```python
from build123d import *

# Parameters (mm, degrees)
SKETCH1_W           = 74.93
SKETCH1_H           = 23.368
BOSS_EXTRUDE1_DEPTH = 20.828
SKETCH2_W           = 5.08
SKETCH2_H           = 10.16
SKETCH2_W_2         = 1.27
BOSS_EXTRUDE2_DEPTH = 7.62
FILLET1_R           = 2.54
FILLET2_R           = 3.81
FILLET3_R           = 2.54
FILLET4_R           = 2.54


with BuildPart() as part:
    # Sketch1 → Boss-Extrude1 (new body)
    with BuildSketch(Plane(origin=(0, 0, 0), x_dir=(1, 0, 0), z_dir=(0, 1, 0))):
        with Locations((37.465, -11.684)):
            Rectangle(SKETCH1_W, SKETCH1_H)
    extrude(amount=BOSS_EXTRUDE1_DEPTH)

    # Sketch2 → Boss-Extrude2 (add)
    with BuildSketch(Plane.ZY):
        with Locations((-2.54, 10.414)):
            Rectangle(SKETCH2_W, SKETCH2_H)
        with Locations((0.635, 10.414)):
            Rectangle(SKETCH2_W_2, SKETCH2_H)
    extrude(amount=BOSS_EXTRUDE2_DEPTH)

    # Fillet1
    fillet1_edges = [part.edges().sort_by_distance(p)[0] for p in [
        (0, 10.414, 0),
        (0, 10.414, 1.27),
    ]]
    fillet(fillet1_edges, radius=FILLET1_R)

    # Fillet2
    fillet2_edges = [part.edges().sort_by_distance(p)[0] for p in [
        (74.93, 20.828, 11.684),
        (0, 20.828, 11.684),
        (74.93, 0, 11.684),
        (0, 0, 11.684),
    ]]
    fillet(fillet2_edges, radius=FILLET2_R)

    # Fillet3
    fillet3_edges = [part.edges().sort_by_distance(p)[0] for p in [
        (37.465, 20.828, 23.368),
        (37.465, 0, 23.368),
        (74.93, 10.414, 23.368),
        (0, 10.414, 23.368),
        (1.115923164, 1.115923164, 23.368),
        (73.814076836, 1.115923164, 23.368),
        (73.814076836, 19.712076836, 23.368),
        (1.115923164, 19.712076836, 23.368),
    ]]
    fillet(fillet3_edges, radius=FILLET3_R)

    # Fillet4
    fillet4_edges = [part.edges().sort_by_distance(p)[0] for p in [
        (0, 16.256, 0),
        (1.115923164, 19.712076836, 0),
        (37.465, 20.828, 0),
        (73.814076836, 19.712076836, 0),
        (74.93, 10.414, 0),
        (73.814076836, 1.115923164, 0),
        (0, 4.572, 0),
        (1.115923164, 1.115923164, 0),
        (37.465, 0, 0),
    ]]
    fillet(fillet4_edges, radius=FILLET4_R)


solid = part.part
```
Check sheet for the modelled part. Datum: model origin and axes. Units: mm. A direction names the side the tool comes from. Coordinates: 2 decimals unless noted, no trailing zeros. Order: outer loops, then holes, each group sorted by start corner. A loop starts at its lowest first (then second) coordinate and runs counter-clockwise, first axis right, second up. Notation, with made-up numbers: (-16.75, 63.5) -> (-4.75, 63.5) arc R31 ccw to (-4.75, 98.5) -> close; hole circle Ø9 at (9, 11.5). An arc over 180 degrees is marked (long way). Write each question's results on one line, items separated by ' | '. Start each with the question number.
1) Set-up check for faces 1 (the face through (-5, 10, 1.27)), 2 (the face through (-4, 10, -5.08)), 3 (the face through (0.724, 4.583, 0.764)), 4 (the face through (0, 10, -4)): record each of +Z, -Z, +X, -X, +Y, -Y from which the full face is reachable in a straight line by a thin tool's end or side.
2) Section check A-A (x = 16.5). Enter the section's corners in (y, z).
3) Material ranges on line 1 along Z through (x, y) = (36, 13.25); line 2 along X through (y, z) = (6.25, 13.75); line 3 along X through (y, z) = (3, 4.25), recorded low to high.
4) Section check C-C (z = 12.5). Enter the section's corners in (x, y), and give its area (3 significant figures).
5) Section check B-B (y = 10.25). Enter the section's corners in (x, z).
6) Section check D-D (z = -1.25). Enter the section's corners in (x, y).
7) Depth check by flat-ended pin: pin 1 (10 mm diameter, centred on x = 31.5, y = 11, fed in from -Z); pin 2 (6 mm diameter, centred on y = 7.5, z = 6, fed in from -X); pin 3 (6.5 mm diameter, centred on y = 13, z = 16, fed in from -X). Enter the tip coordinate at first touch or a pass-through.
Checked values:
1) face 1: +Z, -X, +Y, -Y | face 2: -Z, +X, -X, +Y, -Y | face 3: -Z, -X, -Y | face 4: -Z, +X, +Y, -Y
2) outline: (0, 2.54) arc R2.54 ccw to (2.54, 0) -> (18.29, 0) arc R2.54 ccw to (20.83, 2.54) -> (20.83, 20.83) arc R2.54 ccw to (18.29, 23.37) -> (2.54, 23.37) arc R2.54 ccw to (0, 20.83) -> close
3) line 1: 0 to 23.37 | line 2: 0 to 74.93 | line 3: 0.09 to 74.84
4) outline: (0, 3.81) arc R3.81 ccw to (3.81, 0) -> (71.12, 0) arc R3.81 ccw to (74.93, 3.81) -> (74.93, 17.02) arc R3.81 ccw to (71.12, 20.83) -> (3.81, 20.83) arc R3.81 ccw to (0, 17.02) -> close | area: 1,550 mm²
5) outline: (-7.62, -5.08) -> (0, -5.08) -> (0, -2.54) arc R2.54 cw to (2.54, 0) -> (72.39, 0) arc R2.54 ccw to (74.93, 2.54) -> (74.93, 20.83) arc R2.54 ccw to (72.39, 23.37) -> (2.54, 23.37) arc R2.54 ccw to (0, 20.83) -> (0, 3.81) arc R2.54 cw to (-2.54, 1.27) -> (-7.62, 1.27) -> close
6) outline: (-7.62, 5.33) -> (0.35, 5.33) -> (0.35, 15.49) -> (-7.62, 15.49) -> close
7) pin 1: z = 0 | pin 2: x = -0.13 | pin 3: x = 0
